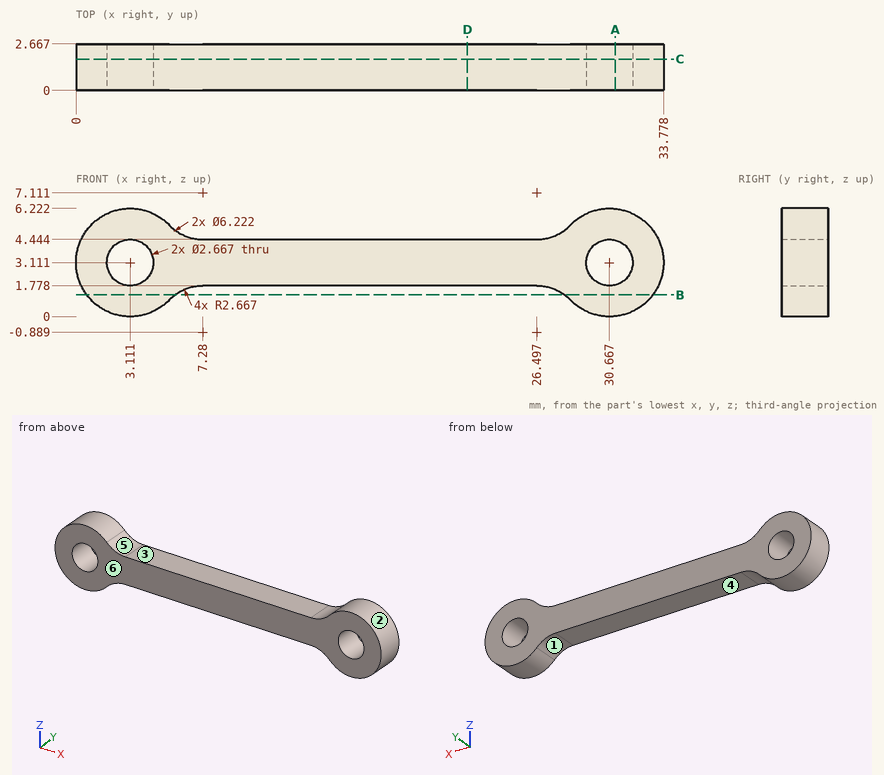
Source: three-view drawing plus pictorial views. Frame: mm from the lowest corner of the part. A direction names the side the tool comes from. Coordinates: 2 decimals unless noted, no trailing zeros. Order: outer loops, then holes, each group sorted by start corner. A loop starts at its lowest first (then second) coordinate and runs counter-clockwise, first axis right, second up.
1) Ray query, probe 1 along X at (y, z) = (0.8, 3) (1 decimal); probe 2 along X at (y, z) = (1.35, 3.5) (1 decimal); probe 3 along Z at (x, y) = (18.5, 1.85) (1 decimal). Return the intervals inside material, ascending.
Result sheet:
probe 1: x = 0 to 1.8, 4.4 to 29.3, 32 to 33.8
probe 2: x = 0 to 1.8, 4.4 to 29.4, 31.9 to 33.8
probe 3: z = 1.8 to 4.4
2) Set-up query: the marked faces 1, 2 and 3. Return all of +Z, -Z, +X, -X, +Y, -Y with unobstructed straight access to the full face (end or side cutting, diameter ignored); none if empty.
Result sheet:
face 1: -Z, +Y, -Y
face 2: +Y, -Y
face 3: +Z, +Y, -Y
3) Section C-C (y = 1.8). Return loops of the section in (x, z) (1 decimal), then the cut area to 3 significant figures.
Result sheet:
outline: (5.4, 1) arc R2.7 cw to (7.3, 1.8) - (26.5, 1.8) arc R2.7 cw to (28.4, 1) arc R3.1 ccw (long way) to (28.4, 5.3) arc R2.7 cw to (26.5, 4.4) - (7.3, 4.4) arc R2.7 cw to (5.4, 5.3) arc R3.1 ccw (long way) to start; hole circle Ø2.7 at (3.1, 3.1); hole circle Ø2.7 at (30.7, 3.1)
area: 108 mm2
4) Section B-B (z = 1.25). Return loops of the section in (x, y).
Result sheet:
outline: (0.62, 0) - (5.69, 0) - (5.69, 2.67) - (0.62, 2.67) - close; (28.09, 0) - (33.16, 0) - (33.16, 2.67) - (28.09, 2.67) - close
5) First-contact query: P1, Ø1, axis at x = 30, y = 0.5, coming from the -Z side (1 decimal); P2, Ø0.8, axis at x = 15, y = 2, coming from the -Z side. Flat tips, straight axial feed; report the tip coordinate or a pass-through.
Result sheet:
P1: stops at z = 0
P2: stops at z = 1.78
6) Section D-D (x = 22.5). Return loops of the section in (y, z) (1 decimal).
Result sheet:
outline: (0, 1.8) - (2.7, 1.8) - (2.7, 4.4) - (0, 4.4) - close
7) Section A-A (x = 31). Return loops of the section in (y, z) (1 decimal).
Result sheet:
outline: (0, 0) - (2.7, 0) - (2.7, 1.8) - (0, 1.8) - close; (0, 4.4) - (2.7, 4.4) - (2.7, 6.2) - (0, 6.2) - close
8) Draft query along X for the marked faces 4, 5 and 6. Return one class per face: released by +X, released by -X, zero draft, split by the parting line, or undercut.
Result sheet:
face 4: undercut
face 5: undercut
face 6: zero draft
